The figure shows three views and two pictorial views of one solid part (mm, origin at its lowest corner). Answer the questions. Round coordinates to 2 decimals unless told otherwise and drop trailing zeros. Write each loop counter-clockwise with the first axis right and the second up, starting at its lowest first coordinate (ties: lowest second). Pieces come first, ordered by that corner, then holes. Notation, with made-up numbers: M 56,16 L 108,16 A13 ccw 108,33 Z; hole C 36.25,-40 d1. An arc over 180 degrees is marked long. One line per item, written item: value. Start each with the question number.
Q1. Find section A-A (y = 32.1). Write down the section's boundary in (x, z).
Q2. Consider probe 1 along Y at (x, z) = (27.2, 4.75); probe 2 along Y at (x, z) = (14.5, 3.4); probe 3 along X at (y, z) = (36, 3.2). Determine where each line is inside the solid, lowest interval first.
Q3. Find section B-B (x = 27.2). Write down the section's boundary in (y, z), and give its area (3 significant figures).
Q4. Find section C-C (z = 3.35). Write down the section's boundary in (x, y).
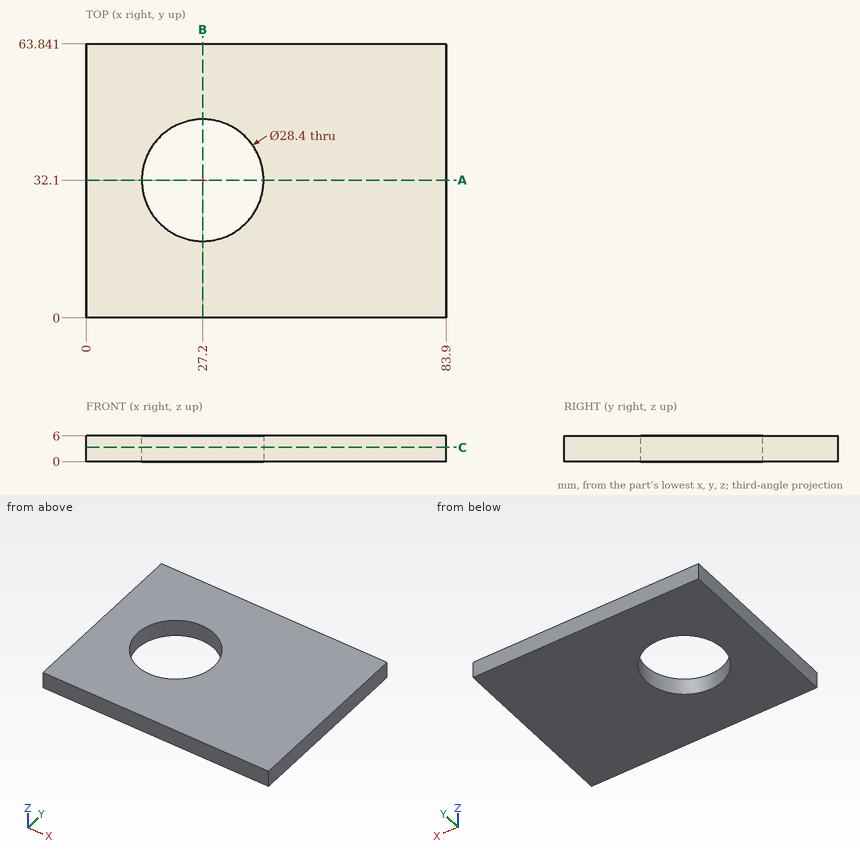
The answers:
1. outline: M 0,0 L 13,0 L 13,6 L 0,6 Z; M 41.4,0 L 83.9,0 L 83.9,6 L 41.4,6 Z
2. probe 1: 0 to 17.9, 46.3 to 63.84
2. probe 2: 0 to 25.75, 38.45 to 63.84
2. probe 3: 0 to 13.55, 40.85 to 83.9
3. outline: M 0,0 L 17.9,0 L 17.9,6 L 0,6 Z; M 46.3,0 L 63.84,0 L 63.84,6 L 46.3,6 Z
3. area: 213 mm2
4. outline: M 0,0 L 83.9,0 L 83.9,63.84 L 0,63.84 Z; hole C 27.2,32.1 d28.4
